Geometry check sheet. Reference: drawing and pictorial views, mm from the part's lowest x, y, z. A direction names the side the tool comes from. Round coordinates to 2 decimals unless told otherwise and drop trailing zeros. Write each loop counter-clockwise with the first axis right and the second up, starting at its lowest first coordinate (ties: lowest second). Pieces come first, ordered by that corner, then holes. Notation, with made-up numbers: M -22,13 L 7,13 A23 cw 7,30 Z; hole C -2,24.5 d7. An arc over 180 degrees is marked long. Answer in a Markdown table with one row per item.
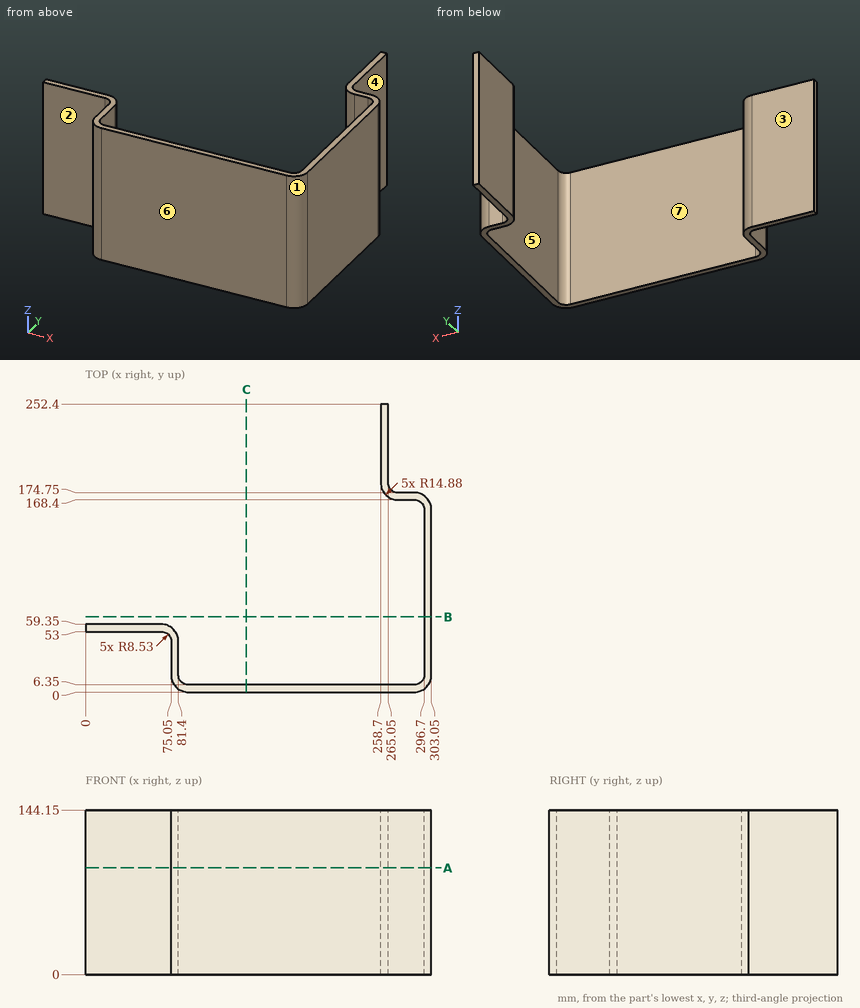
1. Draft check along X on the marked faces 4, 5, 6 and 7. Enter one of: +X half, -X half, draft (parallel to the pull), parting line (faces both ways), or undercut.
Found:
| item | result |
|---|---|
| face 4 | +X half |
| face 5 | undercut |
| face 6 | draft |
| face 7 | undercut |
2. Scan lines: L1, parallel to X at y = 40.5, z = 11; L2, parallel to Y at x = 202.5, z = 60; L3, parallel to X at y = 230.5, z = 20. Record each from-to range of solid material in increasing order.
Found:
| item | result |
|---|---|
| L1 | x = 75.05 to 81.4, 296.7 to 303.05 |
| L2 | y = 0 to 6.35 |
| L3 | x = 258.7 to 265.05 |
3. Section check C-C, the plane x = 141. Record the cut outline in (y, z).
Found:
| item | result |
|---|---|
| outline | M 0,0 L 6.35,0 L 6.35,144.15 L 0,144.15 Z |
4. Section check A-A, the plane z = 93.5. Record the cut outline in (x, y).
Found:
| item | result |
|---|---|
| outline | M 0,53 L 66.52,53 A8.53 cw 75.05,44.47 L 75.05,14.88 A14.88 ccw 89.93,0 L 288.17,0 A14.88 ccw 303.05,14.88 L 303.05,159.87 A14.88 ccw 288.17,174.75 L 273.58,174.75 A8.53 cw 265.05,183.28 L 265.05,252.4 L 258.7,252.4 L 258.7,183.28 A14.88 ccw 273.58,168.4 L 288.17,168.4 A8.53 cw 296.7,159.87 L 296.7,14.88 A8.53 cw 288.17,6.35 L 89.93,6.35 A8.53 cw 81.4,14.88 L 81.4,44.47 A14.88 ccw 66.52,59.35 L 0,59.35 Z |
5. Access from +Z, -Z, +X, -X, +Y, -Y to the whole of each face (thin tool, end or side, straight path). Record for the marked faces 1, 2 and 3.
Found:
| item | result |
|---|---|
| face 1 | +Z, -Z, +X, -Y |
| face 2 | +Z, -Z, -X, -Y |
| face 3 | +Z, -Z, -X, +Y |
6. Section check B-B, the plane y = 66. Record the cut outline in (x, z), and give its area (3 significant figures).
Found:
| item | result |
|---|---|
| outline | M 296.7,0 L 303.05,0 L 303.05,144.15 L 296.7,144.15 Z |
| area | 915 mm2 |
7. Go/stop test with flat-tipped pins: pin 1 (1 mm diameter, centred on y = 92.5, z = 27.5, fed in from -X); pin 2 (23.5 mm diameter, centred on y = 36, z = 52.5, fed in from -X); pin 3 (1 mm diameter, centred on x = 245.5, z = 45, fed in from +Y). Record where each tip stops, or that it passes through.
Found:
| item | result |
|---|---|
| pin 1 | stops at x = 296.7 |
| pin 2 | stops at x = 74.39 |
| pin 3 | stops at y = 6.35 |
